```python
from build123d import *

# Parameters (mm, degrees)
SKETCH2_W           = 39.908935046
SKETCH2_H           = 40.262877017
SKETCH2_R           = 1.4
BOSS_EXTRUDE1_DEPTH = 10
SKETCH5_R           = 3
CUT_EXTRUDE1_DEPTH  = 4
SKETCH6_W           = 14.9
SKETCH6_H           = 30
CUT_EXTRUDE2_DEPTH  = 4
SKETCH9_W           = 10
SKETCH9_H           = 40.262877017
BOSS_EXTRUDE3_DEPTH = 4
SKETCH10_W          = 2
SKETCH10_H          = 30
CUT_EXTRUDE4_DEPTH  = 4
SKETCH11_R          = 2
CUT_EXTRUDE5_DEPTH  = 6


with BuildPart() as part:
    # Sketch2 → Boss-Extrude1 (new body)
    with BuildSketch(Plane.ZY.offset(-34.473625965)):
        with Locations((281.744986803, 328.260975238)):
            Rectangle(SKETCH2_W, SKETCH2_H)
        with Locations((297.699454326, 344.184836729)):
            Circle(SKETCH2_R, mode=Mode.SUBTRACT)
        with Locations((297.699454326, 312.337113746)):
            Circle(SKETCH2_R, mode=Mode.SUBTRACT)
        with Locations((265.79051928, 312.337113746)):
            Circle(SKETCH2_R, mode=Mode.SUBTRACT)
        with Locations((265.79051928, 344.184836729)):
            Circle(SKETCH2_R, mode=Mode.SUBTRACT)
    extrude(amount=BOSS_EXTRUDE1_DEPTH)

    # Sketch5 → Cut-Extrude1 (cut)
    with BuildSketch(Plane.ZY.offset(-24.473625965)):
        with Locations((297.699454326, 344.074881585)):
            Circle(SKETCH5_R)
        with Locations((265.79051928, 312.337113746)):
            Circle(SKETCH5_R)
        with Locations((297.699454326, 312.337113746)):
            Circle(SKETCH5_R)
        with Locations((265.79051928, 344.184836729)):
            Circle(SKETCH5_R)
    extrude(amount=-CUT_EXTRUDE1_DEPTH, mode=Mode.SUBTRACT)

    # Sketch6 → Cut-Extrude2 (cut)
    with BuildSketch(Plane.ZY.offset(-24.473625965)):
        with Locations((294.249454326, 333.392413746)):
            Rectangle(SKETCH6_W, SKETCH6_H)
    extrude(amount=-CUT_EXTRUDE2_DEPTH, mode=Mode.SUBTRACT)

    # Sketch9 → Boss-Extrude3 (add)
    with BuildSketch(Plane.XY.offset(301.699454326)):
        with Locations((29.473625965, 328.260975238)):
            Rectangle(SKETCH9_W, SKETCH9_H)
    extrude(amount=BOSS_EXTRUDE3_DEPTH)

    # Sketch10 → Cut-Extrude4 (cut)
    with BuildSketch(Plane.ZY.offset(-24.473625965)):
        with Locations((302.699454326, 333.392413746)):
            Rectangle(SKETCH10_W, SKETCH10_H)
    extrude(amount=-CUT_EXTRUDE4_DEPTH, mode=Mode.SUBTRACT)

    # Sketch11 → Cut-Extrude5 (cut)
    with BuildSketch(Plane(origin=(0, 348.392413746, 0), x_dir=(1, 0, 0), z_dir=(0, 1, 0))):
        with Locations((29.473625965, -276.79051928)):
            Circle(SKETCH11_R)
    extrude(amount=-CUT_EXTRUDE5_DEPTH, mode=Mode.SUBTRACT)


solid = part.part
```
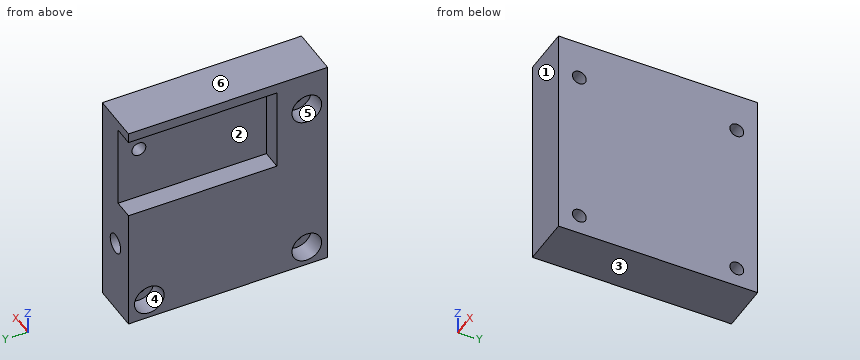
Verification items for the finished model (mm, model axes). Face numbers are marked on the shaded views. A direction names the side the tool comes from. Give positions to 0.01 mm unless a question says otherwise; leave off trailing zeros. Order: outer loops, then holes, each group sorted by start corner. A loop starts at its lowest first (then second) coordinate and runs counter-clockwise, first axis right, second up. Notation, with made-up numbers: (-5, -29) -> (27, -29) arc R32 cw to (27, 9) -> close; hole circle Ø6 at (52.5, 55.5). An arc over 180 degrees is marked (long way). Use a Markdown table: item, result.
1) Tool access check on the marked faces 5 and 6. Record the directions out of +Z, -Z, +X, -X, +Y, -Y that give a thin tool (end or side, any length) a straight path to the whole face; none if there is none.
Results:
| item | result |
|---|---|
| face 5 | -X |
| face 6 | +Z, +X, -X, +Y, -Y |
2) Depth check by flat-ended pin: pin 1 Ø3 at (x, z) = (26.5, 296.5) entering from +Y; pin 2 Ø4.5 at (y, z) = (312.34, 297.7) entering from -X. Enter the tip coordinate at first touch or a pass-through.
Results:
| item | result |
|---|---|
| pin 1 | y = 318.39 |
| pin 2 | x = 28.47 |
3) Section check B-B, the plane z = 290. Record the boundary of the cut face in (x, y), then the cut area to 3 significant figures.
Results:
| item | result |
|---|---|
| outline | (24.47, 308.13) -> (34.47, 308.13) -> (34.47, 348.39) -> (28.47, 348.39) -> (28.47, 318.39) -> (24.47, 318.39) -> close |
| area | 283 mm² |
4) Material ranges on probe 1 along Z at (x, y) = (25, 334); probe 2 along Y at (x, z) = (33.25, 298); probe 3 along Y at (x, z) = (31.5, 266.5), recorded low to high.
Results:
| item | result |
|---|---|
| probe 1 | 261.79 to 286.8, 303.7 to 305.7 |
| probe 2 | 308.13 to 310.97, 313.7 to 342.82, 345.55 to 348.39 |
| probe 3 | 308.13 to 311.13, 313.54 to 342.98, 345.39 to 348.39 |
5) Mould release check, pull along Z, two halves, no side actions. Record for the marked faces 1, 2, 3 and 4: pulls with the +Z half, pulls with the -Z half, needs draft (parallel to the pull), parting line crosses it, or undercut.
Results:
| item | result |
|---|---|
| face 1 | needs draft |
| face 2 | undercut |
| face 3 | pulls with the -Z half |
| face 4 | undercut |
6) Section check A-A, the plane y = 329. Record the boundary of the cut face in (x, z), then the cut area to 3 significant figures.
Results:
| item | result |
|---|---|
| outline | (24.47, 261.79) -> (34.47, 261.79) -> (34.47, 305.7) -> (24.47, 305.7) -> (24.47, 303.7) -> (28.47, 303.7) -> (28.47, 286.8) -> (24.47, 286.8) -> close |
| area | 371 mm² |
7) Section check D-D, the plane z = 277.5. Record the boundary of the cut face in (x, y).
Results:
| item | result |
|---|---|
| outline | (24.47, 308.13) -> (34.47, 308.13) -> (34.47, 348.39) -> (31.34, 348.39) -> (31.34, 342.39) -> (27.6, 342.39) -> (27.6, 348.39) -> (24.47, 348.39) -> close |
8) Section check C-C, the plane x = 30. Record the boundary of the cut face in (y, z), then the cut area to 3 significant figures.
Results:
| item | result |
|---|---|
| outline | (308.13, 261.79) -> (348.39, 261.79) -> (348.39, 274.86) -> (342.39, 274.86) -> (342.39, 278.72) -> (348.39, 278.72) -> (348.39, 305.7) -> (308.13, 305.7) -> close; hole circle Ø2.8 at (312.34, 265.79); hole circle Ø2.8 at (312.34, 297.7); hole circle Ø2.8 at (344.18, 265.79); hole circle Ø2.8 at (344.18, 297.7) |
| area | 1,720 mm² |
